Design review of the part built by this model. Coordinates are the model's own, in mm. Give positions to 0.01 mm unless a question says otherwise; leave off trailing zeros. Write each loop counter-clockwise with the first axis right and the second up, starting at its lowest first coordinate (ties: lowest second). Pieces come first, ordered by that corner, then holes. Notation, with made-up numbers: (8.5, -37) -> (49.5, -37) arc R19 ccw to (49.5, -7) -> close; hole circle Ø1 at (51.25, -24.75). An arc over 180 degrees is marked (long way). Write each question's results on one line, items separated by ' | '. Start each with the question number.
(1) To check wall thickness, follow probe 1 along X at (y, z) = (-1.9, 129); probe 2 along Z at (x, y) = (10.25, -1.65); probe 3 along Z at (x, y) = (14, -1.1). State the ranges of each line that lie inside material, in increasing order.
(2) Take a section at C-C (x = 13.5). State the section outline as (y, z) points, plus the area to 3 significant figures.
(3) Take a section at A-A (z = 49). State the section outline as (x, y) points.
(4) Take a section at B-B (y = -1.3). State the section outline as (x, z) points.
from build123d import *

# Parameters (mm, degrees)
F0_W     = 25.4
F0_H     = 152.4
F1_DEPTH = 2.032


with BuildPart() as f1:
    # F0 (on Front) → F1 (new body)
    with BuildSketch(Plane.XZ):
        with Locations((12.7, 76.2)):
            Rectangle(F0_W, F0_H)
        with BuildLine():
            ThreePointArc((10.16, 30.48), (12.7, 31.0796126628), (15.24, 30.48))
            Line((15.24, 30.48), (15.24, 20.32))
            ThreePointArc((15.24, 20.32), (12.7, 19.7203873372), (10.16, 20.32))
            Line((10.16, 20.32), (10.16, 30.48))
        make_face(mode=Mode.SUBTRACT)
        with BuildLine():
            ThreePointArc((10.16, 55.88), (12.7, 56.4796126628), (15.24, 55.88))
            Line((15.24, 55.88), (15.24, 45.72))
            ThreePointArc((15.24, 45.72), (12.7, 45.1203873372), (10.16, 45.72))
            Line((10.16, 45.72), (10.16, 55.88))
        make_face(mode=Mode.SUBTRACT)
        with BuildLine():
            ThreePointArc((10.16, 81.28), (12.7, 81.8796126628), (15.24, 81.28))
            Line((15.24, 81.28), (15.24, 71.12))
            ThreePointArc((15.24, 71.12), (12.7, 70.5203873372), (10.16, 71.12))
            Line((10.16, 71.12), (10.16, 81.28))
        make_face(mode=Mode.SUBTRACT)
        with BuildLine():
            ThreePointArc((10.16, 106.68), (12.7, 107.2796126628), (15.24, 106.68))
            Line((15.24, 106.68), (15.24, 96.52))
            ThreePointArc((15.24, 96.52), (12.7, 95.9203873372), (10.16, 96.52))
            Line((10.16, 96.52), (10.16, 106.68))
        make_face(mode=Mode.SUBTRACT)
        with BuildLine():
            ThreePointArc((10.16, 132.08), (12.7, 132.6796126628), (15.24, 132.08))
            Line((15.24, 132.08), (15.24, 121.92))
            ThreePointArc((15.24, 121.92), (12.7, 121.3203873372), (10.16, 121.92))
            Line((10.16, 121.92), (10.16, 132.08))
        make_face(mode=Mode.SUBTRACT)
    extrude(amount=F1_DEPTH)


solid = f1.part
Report:
1) probe 1: 0 to 10.16, 15.24 to 25.4 | probe 2: 0 to 20.28, 30.52 to 45.68, 55.92 to 71.08, 81.32 to 96.48, 106.72 to 121.88, 132.12 to 152.4 | probe 3: 0 to 19.87, 30.93 to 45.27, 56.33 to 70.67, 81.73 to 96.07, 107.13 to 121.47, 132.53 to 152.4
2) outline: (-2.03, 0) -> (0, 0) -> (0, 19.78) -> (-2.03, 19.78) -> close; (-2.03, 31.02) -> (0, 31.02) -> (0, 45.18) -> (-2.03, 45.18) -> close; (-2.03, 56.42) -> (0, 56.42) -> (0, 70.58) -> (-2.03, 70.58) -> close; (-2.03, 81.82) -> (0, 81.82) -> (0, 95.98) -> (-2.03, 95.98) -> close; (-2.03, 107.22) -> (0, 107.22) -> (0, 121.38) -> (-2.03, 121.38) -> close; (-2.03, 132.62) -> (0, 132.62) -> (0, 152.4) -> (-2.03, 152.4) -> close | area: 195 mm2
3) outline: (0, -2.03) -> (10.16, -2.03) -> (10.16, 0) -> (0, 0) -> close; (15.24, -2.03) -> (25.4, -2.03) -> (25.4, 0) -> (15.24, 0) -> close
4) outline: (0, 0) -> (25.4, 0) -> (25.4, 152.4) -> (0, 152.4) -> close; hole (10.16, 20.32) arc R5.68 ccw to (15.24, 20.32) -> (15.24, 30.48) arc R5.68 ccw to (10.16, 30.48) -> close; hole (10.16, 45.72) arc R5.68 ccw to (15.24, 45.72) -> (15.24, 55.88) arc R5.68 ccw to (10.16, 55.88) -> close; hole (10.16, 71.12) arc R5.68 ccw to (15.24, 71.12) -> (15.24, 81.28) arc R5.68 ccw to (10.16, 81.28) -> close; hole (10.16, 96.52) arc R5.68 ccw to (15.24, 96.52) -> (15.24, 106.68) arc R5.68 ccw to (10.16, 106.68) -> close; hole (10.16, 121.92) arc R5.68 ccw to (15.24, 121.92) -> (15.24, 132.08) arc R5.68 ccw to (10.16, 132.08) -> close
